Build history of the part. All positions in model axes, mm. A direction names the side the tool comes from. Round coordinates to 2 decimals unless told otherwise and drop trailing zeros. Loops run counter-clockwise (first coordinate to the right, second up) from the corner with the lowest first, then second, coordinate; pieces in that order, holes last. Notation, with made-up numbers: (-36, 39) - (-4, 39) arc R24 cw to (-4, 52) - close; hole circle Ø7 at (30, 75). An arc over 180 degrees is marked (long way). Put each result on its own line as item: value. Start each with the question number.
from build123d import *

# Parameters (mm, degrees)
BOX023_W     = 8
BOX023_H     = 18
BOX023_DEPTH = 9
BOX022_W     = 7
BOX022_H     = 14
BOX022_DEPTH = 8
PAD001_DEPTH = 91
BOX001_W     = 54
BOX001_H     = 87
BOX001_DEPTH = 5
BOX004_W     = 63
BOX004_H     = 91
BOX004_DEPTH = 11


with BuildPart() as cube021:
    # Box023 → Box023 (new body)
    with BuildSketch(Plane(origin=(-23, 18, -11), x_dir=(1, 0, 0), z_dir=(0, 0, 1))):
        with Locations((4, 9)):
            Rectangle(BOX023_W, BOX023_H)
    extrude(amount=BOX023_DEPTH)


with BuildPart() as batterycablehole:
    # Box022 → Box022 (new body)
    with BuildSketch(Plane(origin=(-23, 36, -11), x_dir=(1, 0, 0), z_dir=(0, 0, 1))):
        with Locations((3.5, 7)):
            Rectangle(BOX022_W, BOX022_H)
    extrude(amount=BOX022_DEPTH)

    # Fusion008: union Cube021
    add(cube021.part)


with BuildPart() as batterysliderhole:
    # Sketch001 → Pad001 (new body)
    with BuildSketch(Plane(origin=(46.6, 52, -18.45), x_dir=(-1, 0, 0), z_dir=(0, -1, 0))):
        Polygon((10.546235, -6.448812), (10.546235, -13.448812), (8.546235, -12.448812), (8.546235, -7.448812), align=None)
    extrude(amount=PAD001_DEPTH)


with BuildPart() as batteryhole:
    # Box001 → Box001 (new body)
    with BuildSketch(Plane(origin=(-16, -37, -11), x_dir=(1, 0, 0), z_dir=(0, 0, 1))):
        with Locations((27, 43.5)):
            Rectangle(BOX001_W, BOX001_H)
    extrude(amount=BOX001_DEPTH)


with BuildPart() as cut013:
    # Box004 → Box004 (new body)
    with BuildSketch(Plane(origin=(-25, -39, -14), x_dir=(1, 0, 0), z_dir=(0, 0, 1))):
        with Locations((31.5, 45.5)):
            Rectangle(BOX004_W, BOX004_H)
    extrude(amount=BOX004_DEPTH)

    # Cut004: cut batteryHole
    add(batteryhole.part, mode=Mode.SUBTRACT)

    # Cut012: cut batterySliderHole
    add(batterysliderhole.part, mode=Mode.SUBTRACT)

    # Cut013: cut batteryCableHole
    add(batterycablehole.part, mode=Mode.SUBTRACT)


solid = cut013.part
1) Slice it at B-B, the plane y = 44. Write the cut outline in (x, z).
2) Slice it at A-A, the plane x = 5.5. Write the cut outline in (y, z), and give its area (3 significant figures).
3) Pull direction X, two halves, no side cores. Call faces 4 (the face through (6, 7, -3)), 5 (the face through (38, 6, -5)), 6 (the face through (-15, 27, -5)): pulls with the +X half, pulls with the -X half, needs draft (parallel to the pull), parting line crosses it, or undercut.
4) Slice it at D-D, the plane x = -20. Write the cut outline in (y, z).
5) Drill centre lines: line 1 (Y direction, x = -21.5, z = -8.5); line 2 (Z direction, x = 2, y = 39); line 3 (X direction, y = 38.5, z = -4). Where is each one in solid material? Low to high. Write a range as [from, to].
6) Drop flat-ended pins along their axis: pin 1 Ø4 at (y, z) = (27.5, -7) entering from +X; pin 2 Ø2.5 at (y, z) = (-11.5, -8) entering from +X. Give the stop position or say it passes through.
7) Slice it at C-C, the plane y = 5.5. Write the cut outline in (x, z), and give its area (3 significant figures).
8) Which spindle directions (+Z, -Z, +X, -X, +Y, -Y) get a long thin tool onto all of the face, cutting with end or side? Do faces 1 (the face through (10, -37, -9)), 2 (the face through (6, 7, -14)), 3 (the face through (-19, 18, -7)). Say none if no direction does.
Taken from the geometry:
1. outline: (-25, -14) - (38, -14) - (38, -11.03) - (36.05, -12) - (36.05, -11) - (-23, -11) - (-23, -3) - (-25, -3) - close; (-16, -6) - (36.05, -6) - (36.05, -5) - (38, -5.97) - (38, -3) - (-16, -3) - close
2. outline: (-39, -14) - (52, -14) - (52, -3) - (-39, -3) - close; hole (-37, -11) - (50, -11) - (50, -6) - (-37, -6) - close
2. area: 566 mm2
3. face 4: needs draft
3. face 5: pulls with the +X half
3. face 6: undercut
4. outline: (-39, -14) - (52, -14) - (52, -3) - (50, -3) - (50, -11) - (18, -11) - (18, -3) - (-39, -3) - close
5. line 1: y = [-39, 18], [50, 52]
5. line 2: z = [-14, -11], [-6, -3]
5. line 3: x = [-25, -23], [-16, 38]
6. pin 1: stops at x = 38
6. pin 2: stops at x = -16
7. outline: (-25, -14) - (38, -14) - (38, -11.03) - (36.05, -12) - (36.05, -11) - (-16, -11) - (-16, -6) - (36.05, -6) - (36.05, -5) - (38, -5.97) - (38, -3) - (-25, -3) - close
7. area: 421 mm2
8. face 1: +X
8. face 2: -Z, +X, -X, +Y, -Y
8. face 3: +Z
